Read the model definition and answer for the solid it produces. Units are mm, in the model's axes. A direction names the side the tool comes from. Coordinates: 2 decimals unless noted, no trailing zeros. Write each loop counter-clockwise with the first axis right and the second up, starting at its lowest first coordinate (ties: lowest second). Pieces come first, ordered by that corner, then holes. Notation, with made-up numbers: (-36, -36) -> (-13, -36) arc R7 cw to (-13, -23) -> close; hole circle Ø4 at (-9.5, 59). An arc over 180 degrees is marked (long way). One line per item, written item: value. Start each with the question number.
1. For a pull along Z with two mould halves and no side action, classify faces 4 (the flat face through (-32, 9, 2.54)), 5 (the cylindrical face through (-50.25, 16.02, 7.52)), 6 (the flat face through (-16, 65.405, 12)) as pulls with the +Z half, pulls with the -Z half, needs draft (parallel to the pull), parting line crosses it, or undercut.
2. Find section C-C, the plane y = 31. Write down the section's boundary in (x, z), and give its area (3 significant figures).
3. Find section D-D, the plane x = -56. Write down the section's boundary in (y, z) (1 decimal), and give its area (3 significant figures).
4. Find section A-A, the plane x = -31.75. Write down the section's boundary in (y, z), and give its area (3 significant figures).
5. Find section B-B, the plane z = 16.5. Write down the section's boundary in (x, y) (1 decimal).
6. Consider line 1 along Y through (x, z) = (-6.5, 10) (1 decimal); line 2 along X through (y, z) = (45, 7.5); line 3 along X through (y, z) = (16.3, 8.89). Determine where each line is inside the solid, lowest interval first.
7. For faces 1 (the flat face through (-48, 65.405, 12)), 2 (the flat face through (0, 33, 10)), 3 (the cylindrical face through (-23.526, 16.018, 7.718)), determine the directions among +Z, -Z, +X, -X, +Y, -Y from which every point of the face is accessible in a straight line to the end or side of a thin tool.
8. Given P1, Ø3, axis at x = -44.5, y = 41.5, coming from the +Z side, flat-ended and moving along its own axis, determine where the tip first touches the part or whether it passes through.
```python
from build123d import *

# Parameters (mm, degrees)
SKETCH3_W           = 63.5
SKETCH3_H           = 67.6275
BOSS_EXTRUDE3_DEPTH = 20.32
SKETCH1_W           = 27.94
SKETCH1_H           = 48.26
SKETCH1_W_2         = 59.055
SKETCH1_H_2         = 12.7
CUT_EXTRUDE1_DEPTH  = 17.78
SKETCH4_R           = 2.54
CUT_EXTRUDE2_DEPTH  = 2.2225
SKETCH5_R           = 2.54
CUT_EXTRUDE3_DEPTH  = 2.2225


with BuildPart() as part:
    # Sketch3 → Boss-Extrude3 (new body)
    with BuildSketch(Plane.XY):
        with Locations((-31.75, 33.81375)):
            Rectangle(SKETCH3_W, SKETCH3_H)
    extrude(amount=BOSS_EXTRUDE3_DEPTH)

    # Sketch1 → Cut-Extrude1 (cut)
    with BuildSketch(Plane.XY.offset(20.32)):
        with Locations((-47.3075, 41.275)):
            Rectangle(SKETCH1_W, SKETCH1_H)
        with Locations((-16.1925, 41.275)):
            Rectangle(SKETCH1_W, SKETCH1_H)
        with Locations((-31.75, 8.5725)):
            Rectangle(SKETCH1_W_2, SKETCH1_H_2)
    extrude(amount=-CUT_EXTRUDE1_DEPTH, mode=Mode.SUBTRACT)

    # Sketch4 → Cut-Extrude2 (cut)
    with BuildSketch(Plane.XZ):
        with Locations(Location((-31.75, 10.16, 0), (0, 0, 270))):
            Circle(SKETCH4_R)
    extrude(amount=-CUT_EXTRUDE2_DEPTH, mode=Mode.SUBTRACT)

    # Sketch5 → Cut-Extrude3 (cut)
    with BuildSketch(Plane(origin=(0, 14.9225, 0), x_dir=(-1, 0, 0), z_dir=(0, -1, 0))):
        with Locations(Location((52.3875, -8.89, 0), (0, 0, 90))):
            Circle(SKETCH5_R)
        with Locations(Location((21.2725, -8.89, 0), (0, 0, 90))):
            Circle(SKETCH5_R)
    extrude(amount=-CUT_EXTRUDE3_DEPTH, mode=Mode.SUBTRACT)


solid = part.part
```
Answer block:
1. face 4: pulls with the +Z half
1. face 5: undercut
1. face 6: needs draft
2. outline: (-63.5, 0) -> (0, 0) -> (0, 20.32) -> (-2.22, 20.32) -> (-2.22, 2.54) -> (-30.16, 2.54) -> (-30.16, 20.32) -> (-33.34, 20.32) -> (-33.34, 2.54) -> (-61.28, 2.54) -> (-61.28, 20.32) -> (-63.5, 20.32) -> close
2. area: 297 mm2
3. outline: (0, 0) -> (67.6, 0) -> (67.6, 20.3) -> (65.4, 20.3) -> (65.4, 2.5) -> (17.1, 2.5) -> (17.1, 20.3) -> (14.9, 20.3) -> (14.9, 2.5) -> (2.2, 2.5) -> (2.2, 20.3) -> (0, 20.3) -> close
3. area: 290 mm2
4. outline: (0, 0) -> (67.63, 0) -> (67.63, 20.32) -> (14.92, 20.32) -> (14.92, 2.54) -> (2.22, 2.54) -> (2.22, 7.62) -> (0, 7.62) -> close; (0, 12.7) -> (2.22, 12.7) -> (2.22, 20.32) -> (0, 20.32) -> close
4. area: 1,140 mm2
5. outline: (-63.5, 0) -> (0, 0) -> (0, 67.6) -> (-63.5, 67.6) -> close; hole (-61.3, 2.2) -> (-2.2, 2.2) -> (-2.2, 14.9) -> (-61.3, 14.9) -> close; hole (-61.3, 17.1) -> (-33.3, 17.1) -> (-33.3, 65.4) -> (-61.3, 65.4) -> close; hole (-30.2, 17.1) -> (-2.2, 17.1) -> (-2.2, 65.4) -> (-30.2, 65.4) -> close
6. line 1: y = 0 to 2.2, 14.9 to 17.1, 65.4 to 67.6
6. line 2: x = -63.5 to -61.28, -33.34 to -30.16, -2.22 to 0
6. line 3: x = -63.5 to -54.93, -49.85 to -23.81, -18.73 to 0
7. face 1: +Z
7. face 2: +Z, -Z, +X, +Y, -Y
7. face 3: none
8. P1: stops at z = 2.54
